```python
from build123d import *

# Parameters (mm, degrees)
F0_R     = 7.5
F1_DEPTH = 30
F2_R     = 2.05
F3_DEPTH = 4
F5_R     = 5
F6_DEPTH = 26
F8_R     = 7.5
F8_R_2   = 3.5
F9_DEPTH = 3


with BuildPart() as f1:
    # F0 (on Top) → F1 (new body)
    with BuildSketch(Plane.XY):
        Circle(F0_R)
    extrude(amount=F1_DEPTH)

    # F2 (on Top) → F3 (cut)
    with BuildSketch(Plane.XY):
        Circle(F2_R)
    extrude(amount=F3_DEPTH, mode=Mode.SUBTRACT)

    # F5 (on offset) → F6 (cut, through all)
    with BuildSketch(Plane(origin=(0, 0, 4), x_dir=(1, 0, 0), z_dir=(0, 0, -1))):
        Circle(F5_R)
    extrude(amount=-F6_DEPTH, mode=Mode.SUBTRACT)

    # F8 (on offset) → F9 (cut, through all)
    with BuildSketch(Plane(origin=(0, 0, 3), x_dir=(1, 0, 0), z_dir=(0, 0, -1))):
        Circle(F8_R)
        Circle(F8_R_2, mode=Mode.SUBTRACT)
    extrude(amount=F9_DEPTH, mode=Mode.SUBTRACT)


solid = f1.part
```
Could you check a few things on this model? Use its own coordinates, in mm. A direction names the side the tool comes from. Coordinates: 2 decimals unless noted, no trailing zeros. Loops run counter-clockwise (first coordinate to the right, second up) from the corner with the lowest first, then second, coordinate; pieces in that order, holes last.
1) Which directions (+Z, -Z, +X, -X, +Y, -Y) give clear straight access to the entire face, cutting with the end or side of a thin tool? Please do faces 1 (the face through (-0.1, 2.2, 4)), 2 (the face through (2, -5, 30)), 3 (the face through (3.2, -1.8, 3)).
Reported:
face 1: +Z
face 2: +Z, +X, -X, +Y, -Y
face 3: -Z
2) Thinking about a two-plate mould opening in Y: for faces 4 (the face through (-7.493, 0.33, 16.311)), 5 (the face through (-1.08, 4.88, 16.82)), 6 (the face through (2, -2, 0)), which applies, released by +Y, released by -Y, zero draft, split by the parting line, or undercut?
Reported:
face 4: split by the parting line
face 5: undercut
face 6: zero draft
3) Imagine slicing it at D-D (y = -2.5). List the corners of the cut face in (x, z) for me, and give its area (3 significant figures).
Reported:
outline: (-7.07, 3) - (-2.45, 3) - (-2.45, 0) - (2.45, 0) - (2.45, 3) - (7.07, 3) - (7.07, 30) - (4.33, 30) - (4.33, 4) - (-4.33, 4) - (-4.33, 30) - (-7.07, 30) - close
area: 171 mm2
4) Will these pins go through, and if not, where does the flat tip stop? pin 1 Ø5 at (x, z) = (4, 15.5) entering from +Y; pin 2 Ø6 at (x, z) = (-1, 13.5) entering from -Y; pin 3 Ø1.5 at (x, z) = (-3, 21) entering from -Y; pin 4 Ø4.5 at (x, y) = (0, 0) entering from +Z.
Reported:
pin 1: stops at y = 7.35
pin 2: stops at y = -7.5
pin 3: stops at y = -7.15
pin 4: stops at z = 4
5) Imagine slicing it at C-C (z = 6.5). List the corners of the cut face in (x, y) for me, and give its area (3 significant figures).
Reported:
outline: circle Ø15 at (0, 0); hole circle Ø10 at (0, 0)
area: 98.2 mm2
6) Please list where these lines run through material, in increasing order: line 1 along Y through (x, z) = (0, 12.5); line 2 along X through (y, z) = (0.25, 18.75); line 3 along Z through (x, y) = (3.25, 0.5).
Reported:
line 1: y = -7.5 to -5, 5 to 7.5
line 2: x = -7.5 to -4.99, 4.99 to 7.5
line 3: z = 0 to 4
7) Imagine slicing it at A-A (x = 0). List the corners of the cut face in (y, z) for me.
Reported:
outline: (-7.5, 3) - (-3.5, 3) - (-3.5, 0) - (-2.05, 0) - (-2.05, 4) - (-5, 4) - (-5, 30) - (-7.5, 30) - close; (2.05, 0) - (3.5, 0) - (3.5, 3) - (7.5, 3) - (7.5, 30) - (5, 30) - (5, 4) - (2.05, 4) - close
